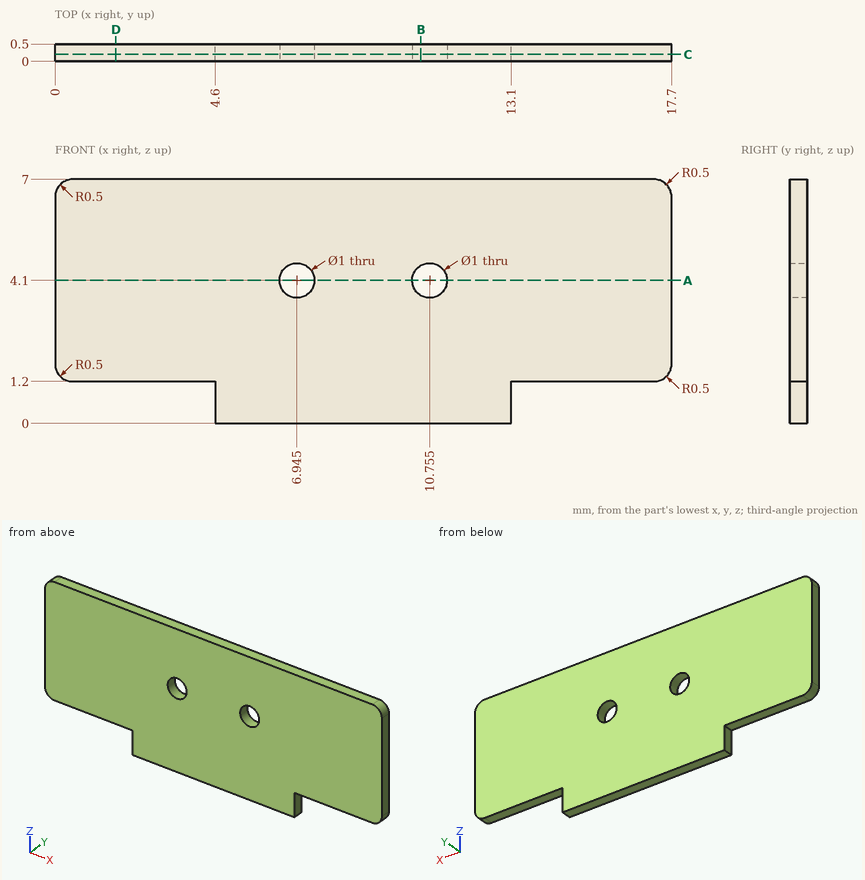
Geometry: see drawing. Coordinates: mm, zero at the bounding-box minimum. Give positions to 0.01 mm unless a question says otherwise; leave off trailing zeros. Order: outer loops, then holes, each group sorted by start corner. A loop starts at its lowest first (then second) coordinate and runs counter-clockwise, first axis right, second up. Notation, with made-up numbers: (20, -6) - (54, -6) arc R25 ccw to (54, 6) - close; hole circle Ø11 at (44.5, 54). An arc over 180 degrees is marked (long way). One line per item, written item: value.
1. Cut plane B-B, the plane x = 10.5. Output: boundary loops of the cut face in (y, z).
Determined:
outline: (0, 0) - (0.5, 0) - (0.5, 3.67) - (0, 3.67) - close; (0, 4.53) - (0.5, 4.53) - (0.5, 7) - (0, 7) - close
2. Cut plane D-D, the plane x = 1.75. Output: boundary loops of the cut face in (y, z), and give its area (3 significant figures).
Determined:
outline: (0, 1.2) - (0.5, 1.2) - (0.5, 7) - (0, 7) - close
area: 2.90 mm2
3. Cut plane C-C, the plane y = 0.2. Output: boundary loops of the cut face in (x, z) (3 decimals).
Determined:
outline: (0, 1.7) arc R0.5 ccw to (0.5, 1.2) - (4.6, 1.2) - (4.6, 0) - (13.1, 0) - (13.1, 1.2) - (17.2, 1.2) arc R0.5 ccw to (17.7, 1.7) - (17.7, 6.5) arc R0.5 ccw to (17.2, 7) - (0.5, 7) arc R0.5 ccw to (0, 6.5) - close; hole circle Ø1 at (6.945, 4.1); hole circle Ø1 at (10.755, 4.1)
4. Line query: probe 1 along X at (y, z) = (0.45, 4.1) (3 decimals); probe 2 along X at (y, z) = (0.4, 4); probe 3 along Z at (x, y) = (15.25, 0.3). Output: solid intervals per line, ascending.
Determined:
probe 1: 0 to 6.445, 7.445 to 10.255, 11.255 to 17.7
probe 2: 0 to 6.46, 7.43 to 10.27, 11.24 to 17.7
probe 3: 1.2 to 7
5. Cut plane A-A, the plane z = 4.1. Output: boundary loops of the cut face in (x, y) (3 decimals).
Determined:
outline: (0, 0) - (6.445, 0) - (6.445, 0.5) - (0, 0.5) - close; (7.445, 0) - (10.255, 0) - (10.255, 0.5) - (7.445, 0.5) - close; (11.255, 0) - (17.7, 0) - (17.7, 0.5) - (11.255, 0.5) - close
